Check sheet for the drawn part. Datum: minimum x, y, z corner. Units: mm. Give positions to 0.01 mm unless a question says otherwise; leave off trailing zeros. Write each loop counter-clockwise with the first axis right and the second up, starting at its lowest first coordinate (ties: lowest second). Pieces come first, ordered by that corner, then holes. Notation, with made-up numbers: (33.5, 74) - (58.5, 74) arc R4 ccw to (58.5, 78) - close; hole circle Ø3 at (-38, -19.5). An arc over 180 degrees is marked (long way). Return JSON: item names as keys, results as strings. Group by question number.
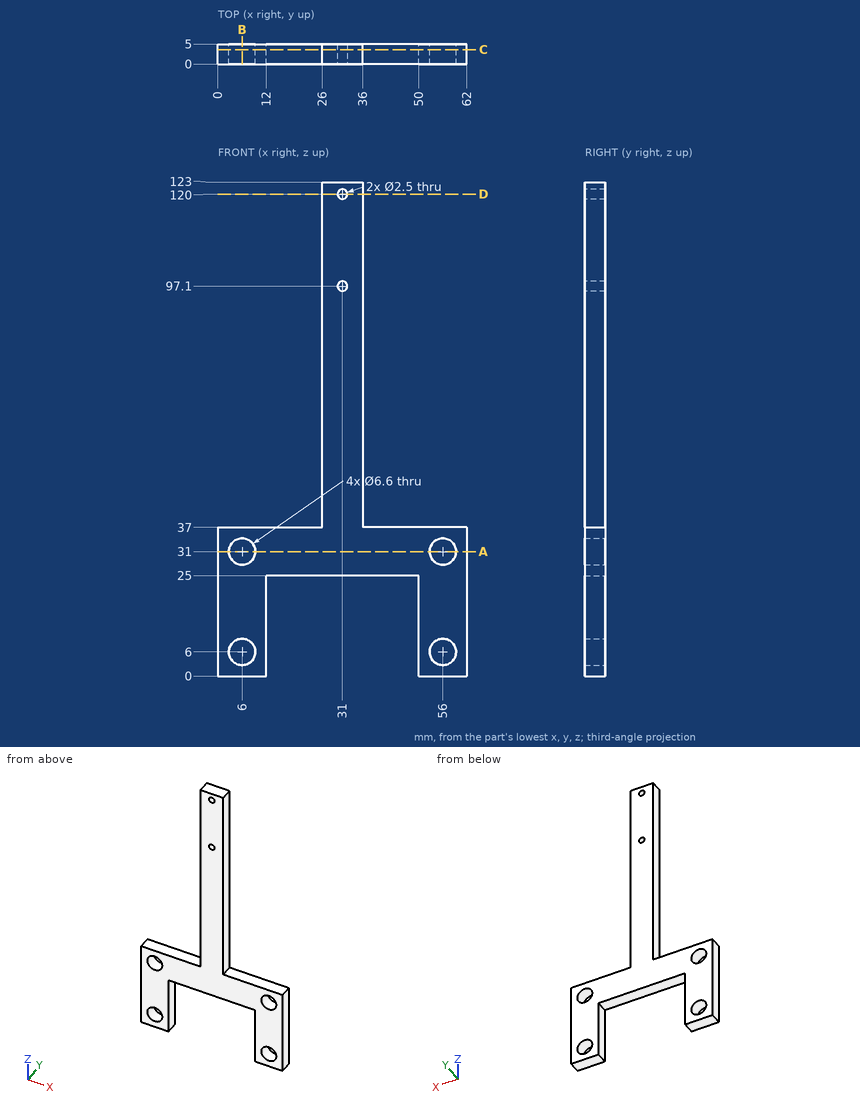
Item 1: Section check A-A on z = 31. Record the cut outline in (x, y).
Item 2: Depth check by flat-ended pin: pin 1 (3 mm diameter, centred on y = 2.5, z = 82, fed in from -X); pin 2 (3 mm diameter, centred on x = 46.5, y = 3.5, fed in from -Z); pin 3 (2.5 mm diameter, centred on x = 14, y = 3, fed in from +Z). Enter the tip coordinate at first touch or a pass-through.
Item 3: Section check B-B on x = 6. Record the cut outline in (y, z), plus the area to 3 significant figures.
Item 4: Section check D-D on z = 120. Record the cut outline in (x, y), plus the area to 3 significant figures.
Item 5: Material ranges on line 1 along X through (y, z) = (3.75, 6); line 2 along Z through (x, y) = (6, 3.6); line 3 along X through (y, z) = (3.65, 31), recorded low to high. Write a range as from..to.
Item 6: Section check C-C on y = 3.6. Record the cut outline in (x, z).
Reply:
{
 "1": {"outline": "(0, 0) - (2.7, 0) - (2.7, 5) - (0, 5) - close; (9.3, 0) - (52.7, 0) - (52.7, 5) - (9.3, 5) - close; (59.3, 0) - (62, 0) - (62, 5) - (59.3, 5) - close"},
 "2": {"pin 1": "x = 26", "pin 2": "z = 25", "pin 3": "z = 37"},
 "3": {"outline": "(0, 0) - (5, 0) - (5, 2.7) - (0, 2.7) - close; (0, 9.3) - (5, 9.3) - (5, 27.7) - (0, 27.7) - close; (0, 34.3) - (5, 34.3) - (5, 37) - (0, 37) - close", "area": "119 mm²"},
 "4": {"outline": "(26, 0) - (29.75, 0) - (29.75, 5) - (26, 5) - close; (32.25, 0) - (36, 0) - (36, 5) - (32.25, 5) - close", "area": "37.5 mm²"},
 "5": {"line 1": "0..2.7, 9.3..12, 50..52.7, 59.3..62", "line 2": "0..2.7, 9.3..27.7, 34.3..37", "line 3": "0..2.7, 9.3..52.7, 59.3..62"},
 "6": {"outline": "(0, 0) - (12, 0) - (12, 25) - (50, 25) - (50, 0) - (62, 0) - (62, 37) - (36, 37) - (36, 123) - (26, 123) - (26, 37) - (0, 37) - close; hole circle Ø6.6 at (6, 6); hole circle Ø6.6 at (6, 31); hole circle Ø2.5 at (31, 97.1); hole circle Ø2.5 at (31, 120); hole circle Ø6.6 at (56, 6); hole circle Ø6.6 at (56, 31)"}
}
